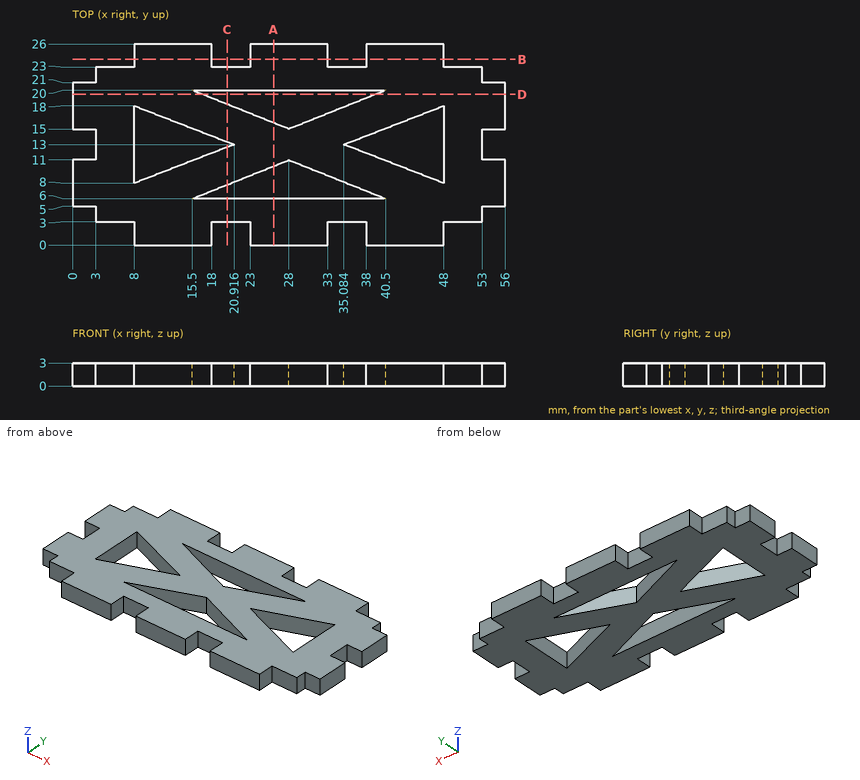
Design review of the part shown in the three views and the two pictorial views. Dimensions are in mm from the part's minimum x, y and z. Give positions to 0.01 mm unless a question says otherwise; leave off trailing zeros. Loops run counter-clockwise (first coordinate to the right, second up) from the corner with the lowest first, then second, coordinate; pieces in that order, holes last. Notation, with made-up numbers: (76.5, 46.5) -> (104.5, 46.5) arc R17 ccw to (104.5, 77.5) -> close; hole circle Ø3 at (40.25, -9.5). An arc over 180 degrees is marked (long way). Put each result on its own line as item: value. Start each with the question number.
1. We need section C-C on x = 20. State the section outline as (y, z) points (1 decimal).
2. We need section D-D on y = 19.5. State the section outline as (x, z) points, then the cut area to 4 significant figures.
3. Wall thickness on probe 1 along X at (y, z) = (23.75, 1.4); probe 2 along Y at (x, z) = (35, 1); probe 3 along Y at (x, z) = (24, 1.5): over which ranges is each line inside the solid? List them lowest first.
4. We need section A-A on x = 26. State the section outline as (y, z) points, then the cut area to 3 significant figures.
5. We need section B-B on y = 24. State the section outline as (x, z) points, then the cut area to 3 significant figures.
6. Clearance check with flat-ended pins moving along their axes: P1, Ø1.5, axis at x = 36.5, z = 0.5, coming from the +Y side; P2, Ø1.5, axis at x = 1.5, z = 1.5, coming from the +Y side; P3, Ø1, axis at y = 13.5, z = 2, coming from the +X side. State where each tip first meets the part, or that it passes through.
Determined:
1. outline: (3, 0) -> (6, 0) -> (6, 3) -> (3, 3) -> close; (7.8, 0) -> (12.6, 0) -> (12.6, 3) -> (7.8, 3) -> close; (13.4, 0) -> (18.2, 0) -> (18.2, 3) -> (13.4, 3) -> close; (20, 0) -> (23, 0) -> (23, 3) -> (20, 3) -> close
2. outline: (0, 0) -> (16.75, 0) -> (16.75, 3) -> (0, 3) -> close; (39.25, 0) -> (56, 0) -> (56, 3) -> (39.25, 3) -> close
2. area: 100.5 mm^2
3. probe 1: 8 to 18, 23 to 33, 38 to 48
3. probe 2: 3 to 6, 8.2 to 17.8, 20 to 23
3. probe 3: 0 to 6, 9.4 to 16.6, 20 to 26
4. outline: (0, 0) -> (6, 0) -> (6, 3) -> (0, 3) -> close; (10.2, 0) -> (15.8, 0) -> (15.8, 3) -> (10.2, 3) -> close; (20, 0) -> (26, 0) -> (26, 3) -> (20, 3) -> close
4. area: 52.8 mm^2
5. outline: (8, 0) -> (18, 0) -> (18, 3) -> (8, 3) -> close; (23, 0) -> (33, 0) -> (33, 3) -> (23, 3) -> close; (38, 0) -> (48, 0) -> (48, 3) -> (38, 3) -> close
5. area: 90.0 mm^2
6. P1: y = 23
6. P2: y = 21
6. P3: x = 53
